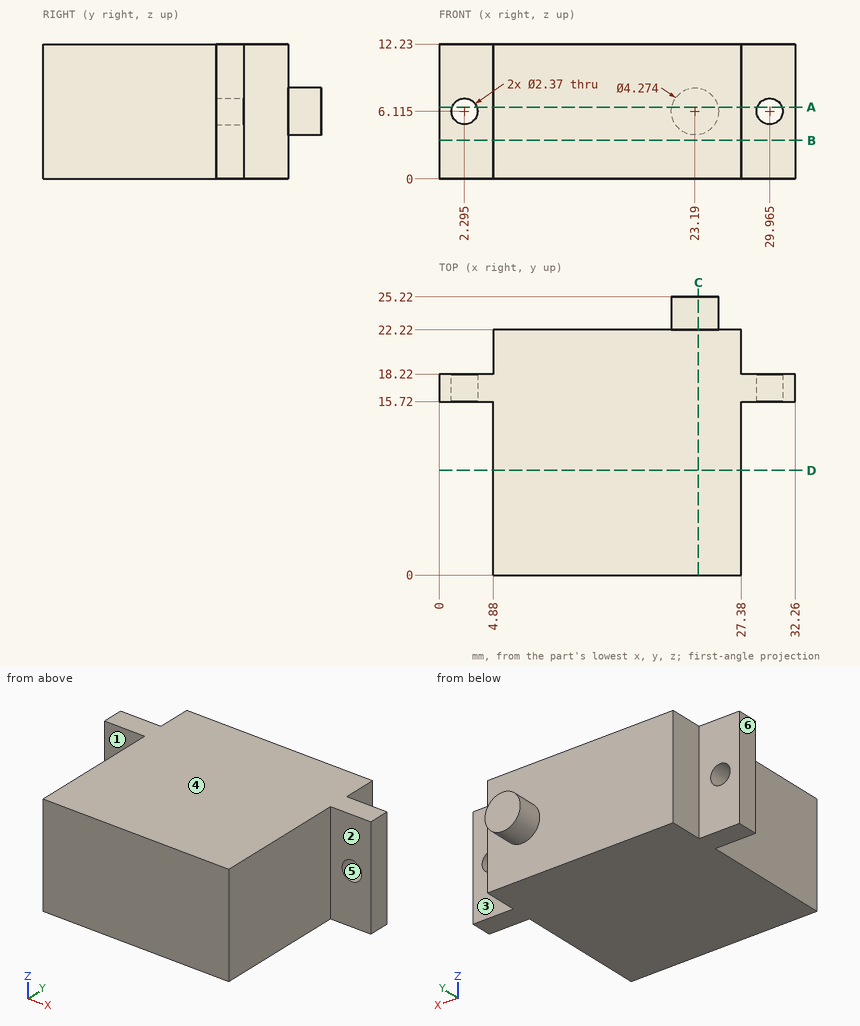
Verification items for this drawing (mm, ordinates from the low corner). A direction names the side the tool comes from. Round coordinates to 2 decimals unless told otherwise and drop trailing zeros. Loops run counter-clockwise (first coordinate to the right, second up) from the corner with the lowest first, then second, coordinate; pieces in that order, holes last. Notation, with made-up numbers: M -2,38.25 L 23,38.25 A19 cw 23,73.25 Z; hole C 84,58 d8. An arc over 180 degrees is marked long. Answer as a JSON object with one key per item and string values.
1. Section check A-A (z = 6.5). Record the boundary of the cut face in (x, y) (1 decimal), plus the area to 3 significant figures.
Reply:
{"outline": "M 0,15.7 L 1.2,15.7 L 1.2,18.2 L 0,18.2 Z; M 3.4,15.7 L 4.9,15.7 L 4.9,0 L 27.4,0 L 27.4,15.7 L 28.8,15.7 L 28.8,18.2 L 27.4,18.2 L 27.4,22.2 L 25.3,22.2 L 25.3,25.2 L 21.1,25.2 L 21.1,22.2 L 4.9,22.2 L 4.9,18.2 L 3.4,18.2 Z; M 31.1,15.7 L 32.3,15.7 L 32.3,18.2 L 31.1,18.2 Z", "area": "526 mm²"}
2. Gauge pin test, flat ends, axial feed: P1, Ø1.5, axis at x = 1, z = 3, coming from the +Y side; P2, Ø4, axis at x = 31, z = 6, coming from the -Y side; P3, Ø4, axis at y = 8.5, z = 2, coming from the +X side. Record the tip position at first contact, or that the pin passes through.
Reply:
{"P1": "stops at y = 18.22", "P2": "stops at y = 15.72", "P3": "stops at x = 27.38"}
3. Access from +Z, -Z, +X, -X, +Y, -Y to the whole of each face (thin tool, end or side, straight path). Record for the marked faces 1, 2 and 3.
Reply:
{"face 1": "+Z, -Z, -X, -Y", "face 2": "+Z, -Z, +X, -Y", "face 3": "+Z, -Z, +X, +Y"}
4. Section check D-D (y = 9.5). Record the boundary of the cut face in (x, z), plus the area to 3 significant figures.
Reply:
{"outline": "M 4.88,0 L 27.38,0 L 27.38,12.23 L 4.88,12.23 Z", "area": "275 mm²"}
5. Mould release check, pull along X, two halves, no side actions. Record for the marked faces 4, 5 and 6: pulls with the +X half, pulls with the -X half, needs draft (parallel to the pull), parting line crosses it, or undercut.
Reply:
{"face 4": "needs draft", "face 5": "undercut", "face 6": "pulls with the -X half"}
6. Scan lines: line 1 (X direction, y = 10.75, z = 5.25); line 2 (Y direction, x = 29, z = 2); line 3 (Y direction, x = 18.5, z = 8.25). Record each from-to range of solid material in increasing order.
Reply:
{"line 1": "x = 4.88 to 27.38", "line 2": "y = 15.72 to 18.22", "line 3": "y = 0 to 22.22"}
7. Section check B-B (z = 3.5). Record the boundary of the cut face in (x, y).
Reply:
{"outline": "M 0,15.72 L 4.88,15.72 L 4.88,0 L 27.38,0 L 27.38,15.72 L 32.26,15.72 L 32.26,18.22 L 27.38,18.22 L 27.38,22.22 L 4.88,22.22 L 4.88,18.22 L 0,18.22 Z"}
8. Section check C-C (x = 23.5). Record the boundary of the cut face in (y, z), plus the area to 3 significant figures.
Reply:
{"outline": "M 0,0 L 22.22,0 L 22.22,4 L 25.22,4 L 25.22,8.23 L 22.22,8.23 L 22.22,12.23 L 0,12.23 Z", "area": "284 mm²"}
